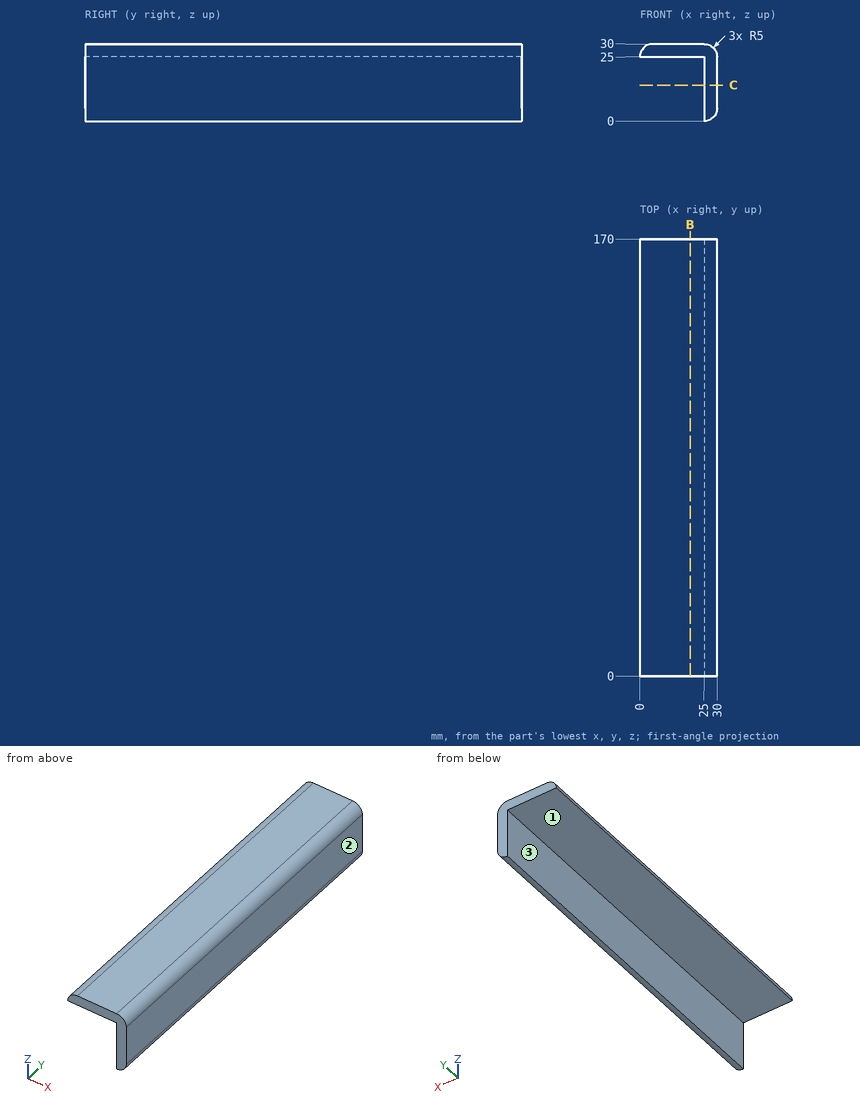
Part print with two shaded views. Sizes in mm from the minimum x, y, z corner. Round coordinates to 2 decimals unless told otherwise and drop trailing zeros. Loops run counter-clockwise (first coordinate to the right, second up) from the corner with the lowest first, then second, coordinate; pieces in that order, holes last.
1. Slice it at C-C (z = 14). Give the cut face in (x, y).
Solutions:
outline: (25, 0) - (30, 0) - (30, 170) - (25, 170) - close
2. Flat gauge pins, fed straight in: pin 1 (12 mm diameter, centred on y = 145, z = 4.5, fed in from -X); pin 2 (7.5 mm diameter, centred on x = 11, y = 120.5, fed in from -Z); pin 3 (1.5 mm diameter, centred on x = 26.5, y = 106, fed in from +Z). Where does each tip first touch, or does it go through?
Solutions:
pin 1: stops at x = 25
pin 2: stops at z = 25
pin 3: stops at z = 29.94
3. Two-plate mould, pull along X, no slides. Class the marked faces 1, 2 and 3: pulls with the +X half, pulls with the -X half, needs draft (parallel to the pull), parting line crosses it, or undercut.
Solutions:
face 1: needs draft
face 2: pulls with the +X half
face 3: pulls with the -X half
4. Drill centre lines: line 1 along X through (y, z) = (118, 21); line 2 along X through (y, z) = (116.5, 1.5). Where is each one in solid material? Low to high.
Solutions:
line 1: x = 25 to 30
line 2: x = 25 to 28.57
5. Slice it at B-B (x = 19.5). Give the cut face in (y, z).
Solutions:
outline: (0, 25) - (170, 25) - (170, 30) - (0, 30) - close
